```python
from build123d import *

# Parameters (mm, degrees)
SKETCH1_R           = 20
BOSS_EXTRUDE1_DEPTH = 40
SKETCH1_7_R         = 8
CUT_EXTRUDE4_DEPTH  = 22
SKETCH3_R           = 10
SKETCH6_W           = 16
SKETCH6_H           = 7
BOSS_EXTRUDE2_DEPTH = 59.518478
CIRPATTERN1_COUNT   = 3
FILLET1_R           = 6


with BuildPart() as part:
    # Sketch1 → Boss-Extrude1 (new body)
    with BuildSketch(Plane(origin=(0, 0, 0), x_dir=(1, 0, 0), z_dir=(0, 1, 0))):
        Circle(SKETCH1_R)
    extrude(amount=BOSS_EXTRUDE1_DEPTH)

    # Sketch1_7 → Cut-Extrude4 (cut)
    with BuildSketch(Plane(origin=(0, 0, 0), x_dir=(1, 0, 0), z_dir=(0, 1, 0))):
        Circle(SKETCH1_7_R)
    extrude(amount=CUT_EXTRUDE4_DEPTH, mode=Mode.SUBTRACT)



with BuildPart() as body_2:
    # Sketch3 → Revolve1 (revolve)
    with BuildSketch(Plane.XY):
        with Locations((-70, 50)):
            Circle(SKETCH3_R)
    revolve(axis=Axis((0, 40, 0), (0, 1, 0)))


with BuildPart() as part_1:
    add(part.part)

    add(body_2.part)  # Boss-Extrude2 merges body 2
    # Sketch6 → Boss-Extrude2 (add)
    with BuildSketch(Plane(origin=(-70, 50, 0), x_dir=(0, 0, 1), z_dir=(-0.894427191, 0.447213595, 0))):
        Rectangle(SKETCH6_W, SKETCH6_H)
    boss_extrude2 = extrude(amount=-BOSS_EXTRUDE2_DEPTH)

    # CirPattern1: Boss-Extrude2 ×3 about axis
    cirpattern1_axis = Axis((0, 0, 0), (0, 1, 0))
    for i in range(1, CIRPATTERN1_COUNT):
        add(boss_extrude2.rotate(cirpattern1_axis, i * 360 / CIRPATTERN1_COUNT))

    # Fillet1
    fillet1_edges = [part_1.edges().sort_by_distance(p)[0] for p in [
        (-20, 40, 0),
    ]]
    fillet(fillet1_edges, radius=FILLET1_R)


solid = part_1.part
```
Check sheet for the modelled part. Datum: model origin and axes. Units: mm. A direction names the side the tool comes from. Give positions to 0.01 mm unless a question says otherwise; leave off trailing zeros. Order: outer loops, then holes, each group sorted by start corner. A loop starts at its lowest first (then second) coordinate and runs counter-clockwise, first axis right, second up. Notation, with made-up numbers: (68.5, -33.5) -> (80.5, -33.5) arc R27 cw to (80.5, -0.5) -> close; hole circle Ø2 at (66, 22.25). An arc over 180 degrees is marked (long way). Return JSON: item names as keys, results as strings.
1. Cross-section at A-A, the plane x = 0. Record the cut outline in (y, z).
From the geometry:
{"outline": "(0, -20) -> (34, -20) arc R6 ccw to (40, -14) -> (40, 14) arc R6 ccw to (34, 20) -> (0, 20) -> (0, 8) -> (22, 8) -> (22, -8) -> (0, -8) -> close; circle Ø20 at (50, -70); circle Ø20 at (50, 70)"}
2. Cross-section at C-C, the plane y = 32. Record the cut outline in (x, z).
From the geometry:
{"outline": "(-41.83, -8) -> (-26.17, -8) -> (-26.17, 8) -> (-41.83, 8) -> close; circle Ø40 at (0, 0); (6.16, -26.67) -> (13.98, -40.22) -> (27.84, -32.22) -> (20.02, -18.67) -> close; (6.16, 26.67) -> (20.02, 18.67) -> (27.84, 32.22) -> (13.98, 40.22) -> close"}
3. Cross-section at B-B, the plane z = 0. Record the cut outline in (x, y).
From the geometry:
{"outline": "(-63.19, 42.68) -> (-20, 21.09) -> (-20, 0) -> (-8, 0) -> (-8, 22) -> (8, 22) -> (8, 0) -> (20, 0) -> (20, 34) arc R6 ccw to (14, 40) -> (-14, 40) arc R6 ccw to (-20, 34) -> (-20, 28.91) -> (-60.06, 48.94) arc R10 ccw (long way) to start; circle Ø20 at (70, 50)"}
4. Mould release check, pull along X, two halves, no side actions. Record for faces 1 (the flat face through (19.672, 38.682, 34.296)), 2 (the flat face through (0, 0, 9)): +X half, -X half, draft (parallel to the pull), parting line (faces both ways), or undercut.
From the geometry:
{"face 1": "undercut", "face 2": "draft"}
5. Go/stop test with flat-tipped pins: P1, Ø6, axis at x = 51, z = 31.5, coming from the -Y side; P2, Ø4, axis at y = 53, z = -12, coming from the +X side; P3, Ø8, axis at y = 42.5, z = 27.5, coming from the +X side. Record where each tip stops, or that it passes through.
From the geometry:
{"P1": "y = 42.91", "P2": "x = 79.17", "P3": "x = 74.94"}
6. Set-up check for faces 3 (the cylindrical face through (-1.73, 10.85, 7.81)), 4 (the flat face through (0, 40, 0)): record each of +Z, -Z, +X, -X, +Y, -Y from which the full face is reachable in a straight line by a thin tool's end or side.
From the geometry:
{"face 3": "-Y", "face 4": "+Y"}
7. Cross-section at D-D, the plane y = 11. Record the cut outline in (x, z), plus the area to 3 significant figures.
From the geometry:
{"outline": "circle Ø40 at (0, 0); hole circle Ø16 at (0, 0)", "area": "1,060 mm^2"}
8. Material ranges on probe 1 along Z at (x, y) = (0, 6.5); probe 2 along Z at (x, y) = (-23, 29.5), recorded low to high. Write a range as [from, to].
From the geometry:
{"probe 1": "[-20, -8], [8, 20]", "probe 2": "[-8, 8]"}
